```python
from build123d import *

# Parameters (mm, degrees)
SKETCH1_W                 = 45
SKETCH1_H                 = 15
BOSS_EXTRUDE1_DEPTH       = 60
SHELL1_T                  = -4
SHELL1_THICKNESS_2_FACE_W = 7
SHELL1_THICKNESS_2_FACE_H = 37
SHELL1_THICKNESS_2_DEPTH  = 2
SKETCH3_W                 = 10
SKETCH3_H                 = 7
CUT_EXTRUDE2_DEPTH        = 4
CUT_EXTRUDE3_REACH        = 67.812
SKETCH4_W                 = 10
SKETCH4_H                 = 10
SKETCH5_W                 = 7.4
SKETCH5_H                 = 7.4
CUT_EXTRUDE4_DEPTH        = 76.374067158
CUT_EXTRUDE5_START        = -1.2
CUT_EXTRUDE5_DEPTH        = 3.6
SKETCH7_R                 = 2.1
CUT_EXTRUDE6_DEPTH        = 123.321298227


with BuildPart() as part:
    # Sketch1 → Boss-Extrude1 (new, symmetric)
    with BuildSketch(Plane(origin=(0, 0, 0), x_dir=(1, 0, 0), z_dir=(0, 1, 0))):
        Rectangle(SKETCH1_W, SKETCH1_H)
    extrude(amount=BOSS_EXTRUDE1_DEPTH, both=True)

    # Shell1
    shell1_openings = [part.faces().sort_by_distance(p)[0] for p in [
        (0, 60, 0),
    ]]
    offset(amount=SHELL1_T, openings=shell1_openings, kind=Kind.INTERSECTION)

    # Shell1 thickness 2 face (on inner face of the shell) → Shell1 thickness 2 (add)
    with BuildSketch(Plane(origin=(0, -56, 0), x_dir=(0, 0, -1), z_dir=(0, -1, 0))):
        Rectangle(SHELL1_THICKNESS_2_FACE_W, SHELL1_THICKNESS_2_FACE_H)
    extrude(amount=-SHELL1_THICKNESS_2_DEPTH)

    # Sketch3 → Cut-Extrude2 (cut)
    with BuildSketch(Plane.XZ.offset(60)):
        Rectangle(SKETCH3_W, SKETCH3_H)
    extrude(amount=-CUT_EXTRUDE2_DEPTH, mode=Mode.SUBTRACT)

    # Sketch4 → Cut-Extrude3 (cut, up to next)
    with BuildSketch(Plane.XY.offset(7.5), mode=Mode.PRIVATE) as cut_extrude3_sk1:
        with Locations((0, 45)):
            Rectangle(SKETCH4_W, SKETCH4_H)
    cut_extrude3_tool1 = extrude(cut_extrude3_sk1.sketch, amount=-CUT_EXTRUDE3_REACH, mode=Mode.PRIVATE) & part.part
    add(cut_extrude3_tool1.solids().sort_by_distance((0, 45, 7.5))[0], mode=Mode.SUBTRACT)

    # Sketch5 → Cut-Extrude4 (cut, through all)
    with BuildSketch(Plane(origin=(22.5, 0, 0), x_dir=(0, 0, -1), z_dir=(1, 0, 0))):
        with Locations((0, 43.5)):
            Rectangle(SKETCH5_W, SKETCH5_H)
    extrude(amount=-CUT_EXTRUDE4_DEPTH, mode=Mode.SUBTRACT)

    # Sketch6 → Cut-Extrude5 (cut)
    with BuildSketch(Plane.XZ.offset(60).offset(CUT_EXTRUDE5_START)):
        Polygon((-15, 4.272391992), (-18.7, 2.136195996), (-18.7, -2.136195996), (-15, -4.272391992), (-11.3, -2.136195996), (-11.3, 2.136195996), align=None)
        Polygon((11.3, 2.136195996), (15, 4.272391992), (18.7, 2.136195996), (18.7, -2.136195996), (15, -4.272391992), (11.3, -2.136195996), align=None)
    extrude(amount=-CUT_EXTRUDE5_DEPTH, mode=Mode.SUBTRACT)

    # Sketch7 → Cut-Extrude6 (cut, through all)
    with BuildSketch(Plane.XZ.offset(60)):
        with Locations(Location((-15, 0, 0), (0, 0, 270))):
            Circle(SKETCH7_R)
        with Locations(Location((15, 0, 0), (0, 0, 90))):
            Circle(SKETCH7_R)
    extrude(amount=-CUT_EXTRUDE6_DEPTH, mode=Mode.SUBTRACT)


solid = part.part
```
The model under review builds one solid part; all positions refer to its coordinate system, in mm. A direction names the side the tool comes from. Coordinates: 2 decimals unless noted, no trailing zeros. Write each loop counter-clockwise with the first axis right and the second up, starting at its lowest first coordinate (ties: lowest second). Pieces come first, ordered by that corner, then holes.
1) Clearance check with flat-ended pins moving along their axes: pin 1 Ø2.5 at (x, z) = (-15, 0) entering from -Y; pin 2 Ø2 at (x, z) = (-9.5, 0) entering from +Y. State where each tip first meets the part, or that it passes through.
2) We need section A-A on y = 22. State the section outline as (x, z) points, then the cut area to 3 significant figures.
3) Machinability: for faces 1 (the face through (-5, 45, 6)), 2 (the face through (0, 54, 3.5)), 3 (the face through (0, 1, 7.5)), 4 (the face through (12.918, -54.608, -0.273)), 5 (the face through (-13, -55.2, -2)), which of the approach directions +Z, -Z, +X, -X, +Y, -Y give a long, thin tool a straight path to every point of the face, cutting with its end or side? Answer none if there is none.
4) To check wall thickness, follow probe 1 along X at (y, z) = (-54.7, 0); probe 2 along Z at (x, y) = (15, -59.5); probe 3 along Z at (x, y) = (-13, -31). State the ranges of each line that lie inside material, in increasing order.
5) We need section B-B on z = 0. Count the separate pieces of the cut face and the enclosed holes in it, then the cut area to 3 significant figures.
6) The part is to be moulded in two halves that separate along Z. For faces 6 (the face through (0, 1, -7.5)), 7 (the face through (-12.918, -59.408, 0.273)), 8 (the face through (0, 60, -5)), 9 (the face through (0, -54, 0)), say which applies: pulls with the +Z half, pulls with the -Z half, needs draft (parallel to the pull), parting line crosses it, or undercut.
Answer list:
1. pin 1: passes through
1. pin 2: stops at y = -54
2. outline: (-22.5, -7.5) - (22.5, -7.5) - (22.5, 7.5) - (-22.5, 7.5) - close; hole (-18.5, -3.5) - (18.5, -3.5) - (18.5, 3.5) - (-18.5, 3.5) - close
2. area: 416 mm2
3. face 1: +Z
3. face 2: +Y
3. face 3: +Z, +X, -X, +Y, -Y
3. face 4: +Y, -Y
3. face 5: none
4. probe 1: x = -22.5 to -17.1, -12.9 to 12.9, 17.1 to 22.5
4. probe 2: z = -7.5 to -2.1, 2.1 to 7.5
4. probe 3: z = -7.5 to -3.5, 3.5 to 7.5
5. separate pieces: 5
5. enclosed holes: 0
5. area: 1,010 mm2
6. face 6: pulls with the -Z half
6. face 7: undercut
6. face 8: needs draft
6. face 9: undercut
